Can you work these out from the model? Positions are in its coordinate system, mm. A direction names the side the tool comes from. Round coordinates to 2 decimals unless told otherwise and drop trailing zeros. Order: outer loops, then holes, each group sorted by start corner. A loop starts at its lowest first (then second) coordinate and runs counter-clockwise, first axis right, second up. Notation, with made-up numbers: (89.5, -26) -> (97.5, -26) arc R27 cw to (97.5, 7) -> close; hole circle Ø10 at (46, 51). An arc over 180 degrees is marked (long way). Use a Markdown table: item, result. Add a question column.
Q1. I need wall thicknesses on line 1 along Y through (x, z) = (12.5, 1.2); line 2 along Y through (x, z) = (9.5, 1.7); line 3 along Y through (x, z) = (19.25, 2.85). Which ranges of each line are inside material? Lowest first, please. Write a range as [from, to].
Q2. We'd pull the mould along X, two halves only. Please class faces 1 (the face through (12.17, -127.47, 1.52)), 2 (the face through (-1.27, -0.97, 1.48)), 3 (the face through (10, -48, 3)), 4 (the face through (7, -134, 1)): +X half, -X half, draft (parallel to the pull), parting line (faces both ways), or undercut.
Q3. If we section it at B-B on z = 0.6: List the corners of the cut face in (x, y) for me.
Q4. If we section it at A-A on x = 12.5: List the corners of the cut face in (y, z) for me, plus the area to 3 significant figures.
Q5. For faces 5 (the face through (22.477, -63.166, 1.479)), 6 (the face through (5, -106, 1)), which set-ups out of +Z, -Z, +X, -X, +Y, -Y let a thin tool reach every point of the face, with its end or its side?
Q6. If we section it at D-D on x = 0: List the corners of the cut face in (y, z) for me.
Q7. I'm going to push a flat-ended pin straight in: pin 1 Ø3 at (x, y) = (3, -43.5) entering from -Z. Where does the tip first touch, or does it pass through?
Q8. If we section it at C-C on y = 0: List the corners of the cut face in (x, z) for me, plus the area to 3 significant figures.
```python
from build123d import *
from OCP.BRepFilletAPI import BRepFilletAPI_MakeChamfer

# Parameters (mm, degrees)
SKETCH_1_W          = 30
SKETCH_1_H          = 140
SKETCH_1_R          = 1.6
EXTRUDE_1_DEPTH     = 3
CUT_EXTRUDE_3_REACH = 139.328
SKETCH_4_W          = 5
SKETCH_4_H          = 55
CHAMFER_1_SIZE      = 2.5
CUT_EXTRUDE_4_REACH = 139.328
SKETCH_5_R          = 2.55
EXTRUDE_5_DEPTH     = 3
EXTRUDE_2_DEPTH     = 3
FILLET_2_R          = 65
FILLET_3_R          = 115
FILLET_4_R          = 5
CUT_EXTRUDE_START   = -3
CUT_EXTRUDE_6_DEPTH = 3
CHAMFER_2_SIZE      = 3
CHAMFER_2_SIZE2     = 2.894908666


# Read off the part's stored shape, not the designer's step: 切除-拉伸6
with BuildPart() as part:
    # 草图1 → 凸台-拉伸1 (new body)
    with BuildSketch(Plane.XY):
        with Locations((10, -65)):
            Rectangle(SKETCH_1_W, SKETCH_1_H)
        Circle(SKETCH_1_R, mode=Mode.SUBTRACT)
        with Locations((20, 0)):
            Circle(SKETCH_1_R, mode=Mode.SUBTRACT)
    extrude(amount=EXTRUDE_1_DEPTH)

    # 草图4 → 切除-拉伸3 (cut, up to next)
    with BuildSketch(Plane.XY.offset(3), mode=Mode.PRIVATE) as cut_extrude_3_sk1:
        with Locations((-2.5, -107.5)):
            Rectangle(SKETCH_4_W, SKETCH_4_H)
    cut_extrude_3_tool1 = extrude(cut_extrude_3_sk1.sketch, amount=-CUT_EXTRUDE_3_REACH, mode=Mode.PRIVATE) & part.part
    add(cut_extrude_3_tool1.solids().sort_by_distance((-2.5, -107.5, 3))[0], mode=Mode.SUBTRACT)

    # 倒角1
    chamfer_1_edges = [part.edges().sort_by_distance(p)[0] for p in [
        (-5, -80, 1.5),
    ]]
    chamfer(chamfer_1_edges, length=CHAMFER_1_SIZE)

    # 草图5 → 切除-拉伸4 (cut, up to next)
    with BuildSketch(Plane.XY.offset(3), mode=Mode.PRIVATE) as cut_extrude_4_sk1:
        with Locations((12.5, -130)):
            Circle(SKETCH_5_R)
    cut_extrude_4_tool1 = extrude(cut_extrude_4_sk1.sketch, amount=-CUT_EXTRUDE_4_REACH, mode=Mode.PRIVATE) & part.part
    add(cut_extrude_4_tool1.solids().sort_by_distance((12.5, -130, 3))[0], mode=Mode.SUBTRACT)

    # 草图9 → 凸台-拉伸5 (add)
    with BuildSketch(Plane(origin=(0, 0, 0), x_dir=(-1, 0, 0), z_dir=(0, 0, -1))):
        Polygon((5, -77.5), (0, -107.5), (0, -80), (2.5, -80), align=None)
    extrude(amount=-EXTRUDE_5_DEPTH)

    # 草图11 → 拉伸-薄壁2 (add)
    with BuildSketch(Plane.XY.offset(3)):
        Polygon((19.5, -67.916286439), (19.5, -61.710608008), (19.5, -3.420169007), (16.5, -3.420169007), (16.5, -61.710608008), (16.5, -67.916286439), align=None)
    extrude(amount=-EXTRUDE_2_DEPTH)

    # 圆角2
    fillet_2_edges = [part.edges().sort_by_distance(p)[0] for p in [
        (-5, -77.5, 1.5),
    ]]
    fillet(fillet_2_edges, radius=FILLET_2_R)

    # 圆角3
    fillet_3_edges = [part.edges().sort_by_distance(p)[0] for p in [
        (0, -107.5, 1.5),
    ]]
    fillet(fillet_3_edges, radius=FILLET_3_R)

    # 圆角4
    fillet_4_edges = [part.edges().sort_by_distance(p)[0] for p in [
        (0, -135, 1.5),
    ]]
    fillet(fillet_4_edges, radius=FILLET_4_R)

    # 切除-拉伸6 outline → 切除-拉伸6 (cut)
    with BuildSketch(Plane.XY.offset(3).offset(CUT_EXTRUDE_START)):
        with BuildLine():
            ThreePointArc((19.996578854, -130.184931767), (18.469534635, -133.600323516), (15, -135))
            Line((15, -135), (25, -135))
            Line((25, -135), (25, 5))
            Line((25, 5), (19.996578854, -130.184931767))
        make_face()
        with BuildLine():
            ThreePointArc((10, -135), (6.464466094, -133.535533906), (5, -130))
            Line((5, -130), (5, -82.212778368))
            ThreePointArc((5, -82.212778368), (2.962270532, -62.17737686), (-3.067466378, -42.962488681))
            ThreePointArc((-3.067466378, -42.962488681), (-4.511868965, -38.359628786), (-5, -33.560217765))
            Line((-5, -33.560217765), (-5, -72.120435531))
            ThreePointArc((-5, -72.120435531), (-4.778523942, -77.481670081), (-4.115605049, -82.806369705))
            Line((-4.115605049, -82.806369705), (-1.564698759, -98.111807444))
            ThreePointArc((-1.564698759, -98.111807444), (-0.391842257, -107.532429856), (0, -117.017690984))
            Line((0, -117.017690984), (0, -130))
            ThreePointArc((0, -130), (1.464466094, -133.535533906), (5, -135))
            Line((5, -135), (10, -135))
        make_face()
    extrude(amount=CUT_EXTRUDE_6_DEPTH, mode=Mode.SUBTRACT)

    # 倒角2: one chamfer whose edges measure the first distance from different faces: ONE call of the kernel's chamfer builder (chamfer() names one face for all edges)
    chamfer_2_edges_1 = [part.edges().sort_by_distance(p)[0] for p in [
        (-5, 5, 1.5),
    ]]
    chamfer_2_edges_2 = [part.edges().sort_by_distance(p)[0] for p in [
        (25, 5, 1.5),
    ]]
    chamfer_2_side_2 = [part.faces().sort_by_distance(p)[0] for p in [
        (22.498289427, -62.592465884, 1.5),
    ]]
    chamfer_2 = BRepFilletAPI_MakeChamfer(part.part.solid().wrapped)
    for e in chamfer_2_edges_1:
        chamfer_2.Add(CHAMFER_2_SIZE, e.wrapped)
    for e in chamfer_2_edges_2:
        chamfer_2.Add(CHAMFER_2_SIZE, CHAMFER_2_SIZE2, e.wrapped, chamfer_2_side_2[0].wrapped)  # the first distance lies on this face
    add(Compound.cast(chamfer_2.Shape()), mode=Mode.REPLACE)


solid = part.part
```
Answer below:
| question | item | result |
|---|---|---|
| 1 | line 1 | [-135, -132.55], [-127.45, 5] |
| 1 | line 2 | [-134.97, 5] |
| 1 | line 3 | [-132.63, -1.41], [1.41, 5] |
| 2 | face 1 | undercut |
| 2 | face 2 | undercut |
| 2 | face 3 | draft |
| 2 | face 4 | -X half |
| 3 | outline | (-5, -33.56) arc R23.84 ccw to (-3.07, -42.96) arc R99.52 cw to (5, -82.21) -> (5, -130) arc R5 ccw to (10, -135) -> (15, -135) arc R5 ccw to (20, -130.18) -> (24.89, 2) -> (22.11, 5) -> (-2, 5) -> (-5, 2) -> close; hole circle Ø3.2 at (0, 0); hole circle Ø5.1 at (12.5, -130); hole circle Ø3.2 at (20, 0) |
| 4 | outline | (-135, 0) -> (-132.55, 0) -> (-132.55, 3) -> (-135, 3) -> close; (-127.45, 0) -> (5, 0) -> (5, 3) -> (-127.45, 3) -> close |
| 4 | area | 405 mm² |
| 5 | face 5 | +Z, -Z, +X, -Y |
| 5 | face 6 | +Z, -Z, -X, -Y |
| 6 | outline | (-51.07, 0) -> (-1.6, 0) -> (-1.6, 3) -> (-51.07, 3) -> close; (1.6, 0) -> (5, 0) -> (5, 3) -> (1.6, 3) -> close |
| 7 | pin 1 | z = 0 |
| 8 | outline | (-5, 0) -> (-1.6, 0) -> (-1.6, 3) -> (-5, 3) -> close; (1.6, 0) -> (18.4, 0) -> (18.4, 3) -> (1.6, 3) -> close; (21.6, 0) -> (24.81, 0) -> (24.81, 3) -> (21.6, 3) -> close |
| 8 | area | 70.2 mm² |
